from build123d import *

# Parameters (mm, degrees)
F0_W     = 61.199996
F0_H     = 127.500012
F1_DEPTH = 12.5
F2_R     = 7.484062


with BuildPart() as f1:
    # F0 (on Front) → F1 (new body, symmetric)
    with BuildSketch(Plane.XZ):
        Rectangle(F0_W, F0_H)
    extrude(amount=F1_DEPTH, both=True)

    # F2
    f2_edges = [f1.edges().sort_by_distance(p)[0] for p in [
        (-30.599998, 0, 63.750006),
        (0, -12.5, 63.750006),
        (30.599998, 0, 63.750006),
        (0, 12.5, 63.750006),
        (30.599998, -12.5, 0),
        (30.599998, 12.5, 0),
        (0, -12.5, -63.750006),
        (30.599998, 0, -63.750006),
        (0, 12.5, -63.750006),
        (-30.599998, 0, -63.750006),
    ]]
    fillet(f2_edges, radius=F2_R)


solid = f1.part
Here's how the part is built. I have some questions about the finished solid (model axes, mm). Round coordinates to 2 decimals unless told otherwise and drop trailing zeros. Write each loop counter-clockwise with the first axis right and the second up, starting at its lowest first coordinate (ties: lowest second). Pieces come first, ordered by that corner, then holes. Notation, with made-up numbers: (4.25, 37.25) -> (18.25, 37.25) arc R17 ccw to (18.25, 68.25) -> close; hole circle Ø8 at (5, 53.5). An arc over 180 degrees is marked (long way). One line per item, written item: value.
1) I'm going to push a flat-ended pin straight in: pin 1 Ø1.5 at (x, y) = (-8.5, -7) entering from -Z. Where does the tip first touch, or does it pass through?
Filled sheet:
pin 1: stops at z = -63.65
2) Suppose I cut it at B-B on x = -21. List the corners of the cut face in (y, z) for me.
Filled sheet:
outline: (-12.5, -56.27) arc R7.48 ccw to (-5.02, -63.75) -> (5.02, -63.75) arc R7.48 ccw to (12.5, -56.27) -> (12.5, 56.27) arc R7.48 ccw to (5.02, 63.75) -> (-5.02, 63.75) arc R7.48 ccw to (-12.5, 56.27) -> close
3) Suppose I cut it at C-C on y = 9.5. List the corners of the cut face in (x, z) for me, plus the area to 3 significant figures.
Filled sheet:
outline: (-30.6, -56.27) arc R7.48 ccw to (-27.6, -62.26) -> (23.12, -62.26) arc R5.99 ccw to (29.11, -56.27) -> (29.11, 56.27) arc R5.99 ccw to (23.12, 62.26) -> (-27.6, 62.26) arc R7.48 ccw to (-30.6, 56.27) -> close
area: 7,410 mm2
4) Suppose I cut it at A-A on z = -23. List the corners of the cut face in (x, y) for me.
Filled sheet:
outline: (-30.6, -12.5) -> (23.12, -12.5) arc R7.48 ccw to (30.6, -5.02) -> (30.6, 5.02) arc R7.48 ccw to (23.12, 12.5) -> (-30.6, 12.5) -> close
5) If I drill on line 1 (X direction, y = -5.25, z = 51.5); line 2 (X direction, y = -8.5, z = -17.5); line 3 (Z direction, x = 0.5, y = -5.5), over which ranges is the centre line in solid material (lowest first)? Write a range as [from, to].
Filled sheet:
line 1: x = [-30.6, 30.6]
line 2: x = [-30.6, 29.74]
line 3: z = [-63.73, 63.73]
